```python
from build123d import *

# Parameters (mm, degrees)
SKETCH1_W           = 28.3
SKETCH1_H           = 51.75
SKETCH1_R           = 1.5
BOSS_EXTRUDE1_DEPTH = 1.5
FILLET1_R           = 3
SKETCH2_W           = 18
SKETCH2_H           = 26
BOSS_EXTRUDE2_DEPTH = 3.2
SKETCH3_W           = 7.45
SKETCH3_H           = 5.6
BOSS_EXTRUDE3_DEPTH = 2.5


with BuildPart() as part:
    # Sketch1 → Boss-Extrude1 (new body)
    with BuildSketch(Plane.XY):
        with Locations((14.15, 25.875)):
            Rectangle(SKETCH1_W, SKETCH1_H)
        with Locations((2.65, 49.4)):
            Circle(SKETCH1_R, mode=Mode.SUBTRACT)
        with Locations((25.65, 49.4)):
            Circle(SKETCH1_R, mode=Mode.SUBTRACT)
        with Locations((2.65, 2.85)):
            Circle(SKETCH1_R, mode=Mode.SUBTRACT)
        with Locations((25.65, 2.85)):
            Circle(SKETCH1_R, mode=Mode.SUBTRACT)
    extrude(amount=BOSS_EXTRUDE1_DEPTH)

    # Fillet1
    fillet1_edges = [part.edges().sort_by_distance(p)[0] for p in [
        (0, 51.75, 0.75),
        (28.3, 51.75, 0.75),
        (28.3, 0, 0.75),
        (0, 0, 0.75),
    ]]
    fillet(fillet1_edges, radius=FILLET1_R)

    # Sketch2 → Boss-Extrude2 (add)
    with BuildSketch(Plane.XY.offset(1.5)):
        with Locations((14.15, 13.8)):
            Rectangle(SKETCH2_W, SKETCH2_H)
    extrude(amount=BOSS_EXTRUDE2_DEPTH)

    # Sketch3 → Boss-Extrude3 (add)
    with BuildSketch(Plane.XY.offset(1.5)):
        with Locations((14.15, 49.15)):
            Rectangle(SKETCH3_W, SKETCH3_H)
    extrude(amount=BOSS_EXTRUDE3_DEPTH)


solid = part.part
```
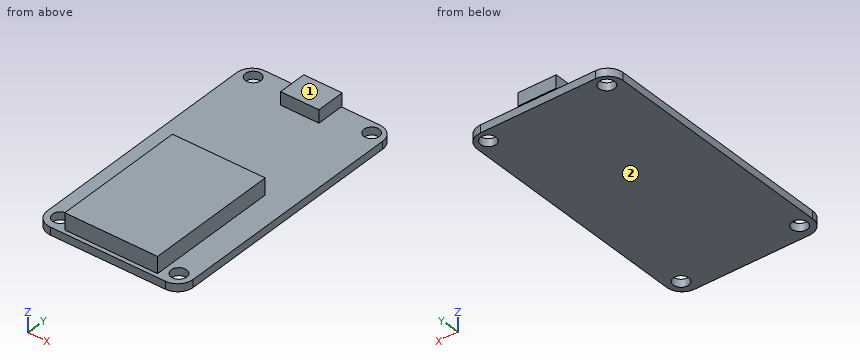
CAD build for the part. Positions are in the model's coordinates, mm. Face numbers are marked on the shaded views. A direction names the side the tool comes from. Coordinates: 2 decimals unless noted, no trailing zeros. Write each loop counter-clockwise with the first axis right and the second up, starting at its lowest first coordinate (ties: lowest second). Pieces come first, ordered by that corner, then holes. Notation, with made-up numbers: (-17, 6) -> (23, 6) arc R19 cw to (23, 32) -> close; hole circle Ø6 at (61, 53.25). An arc over 180 degrees is marked (long way). Use CSV: the item, a comma, the result in double quotes. Start each with the question number.
Item 1: Band-saw the part on C-C, the plane y = 49.4. Write the cut outline in (x, z) (3 decimals), plus the area to 3 significant figures.
Item 2: Drop flat-ended pins along their axis: P1, Ø5, axis at x = 2.65, y = 49.4, coming from the +Z side; P2, Ø1.2, axis at y = 50, z = 2.5, coming from the -X side (3 decimals); P3, Ø1.6, axis at x = 10, z = 3.5, coming from the -Y side. Give the stop position or say it passes through.
Item 3: Wall check: probe 1 along Y at (x, z) = (12, 3.7); probe 2 along Y at (x, z) = (2.65, 0.3); probe 3 along Y at (x, z) = (9, 2.25). Give the ranges that are in metal, low to high.
Item 4: Band-saw the part on A-A, the plane z = 3.1. Write the cut outline in (x, y) (3 decimals), plus the area to 3 significant figures.
Item 5: Band-saw the part on B-B, the plane x = 21. Write the cut outline in (y, z).
Item 6: Band-saw the part on D-D, the plane y = 5.5. Write the cut outline in (x, z), plus the area to 3 significant figures.
Item 7: Tool access for the marked faces 1 and 2: list every direction of +Z, -Z, +X, -X, +Y, -Y with a clear straight run to the whole face (end or side of a thin tool).
Response values:
1,outline,"(0.071, 0) -> (1.15, 0) -> (1.15, 1.5) -> (0.071, 1.5) -> close; (4.15, 0) -> (24.15, 0) -> (24.15, 1.5) -> (17.875, 1.5) -> (17.875, 4) -> (10.425, 4) -> (10.425, 1.5) -> (4.15, 1.5) -> close; (27.15, 0) -> (28.229, 0) -> (28.229, 1.5) -> (27.15, 1.5) -> close"
1,area,"51.9 mm2"
2,P1,"stops at z = 1.5"
2,P2,"stops at x = 10.425"
2,P3,"stops at y = 0.8"
3,probe 1,"y = 0.8 to 26.8, 46.35 to 51.95"
3,probe 2,"y = 0.02 to 1.35, 4.35 to 47.9, 50.9 to 51.73"
3,probe 3,"y = 0.8 to 26.8"
4,outline,"(5.15, 0.8) -> (23.15, 0.8) -> (23.15, 26.8) -> (5.15, 26.8) -> close; (10.425, 46.35) -> (17.875, 46.35) -> (17.875, 51.95) -> (10.425, 51.95) -> close"
4,area,"510 mm2"
5,outline,"(0, 0) -> (51.75, 0) -> (51.75, 1.5) -> (26.8, 1.5) -> (26.8, 4.7) -> (0.8, 4.7) -> (0.8, 1.5) -> (0, 1.5) -> close"
6,outline,"(0, 0) -> (28.3, 0) -> (28.3, 1.5) -> (23.15, 1.5) -> (23.15, 4.7) -> (5.15, 4.7) -> (5.15, 1.5) -> (0, 1.5) -> close"
6,area,"100 mm2"
7,face 1,"+Z, +X, -X, +Y"
7,face 2,"-Z, +X, -X, +Y, -Y"
